```python
from build123d import *

# Parameters (mm, degrees)
BOSS_EXTRUDE1_DEPTH = 10
SKETCH2_R           = 2
CUT_EXTRUDE1_DEPTH  = 127.711975624
FILLET1_R           = 2
L_EK1_SCALE         = 2
L_EK2_SCALE         = 0.4


with BuildPart() as part:
    # Sketch1 → Boss-Extrude1 (new body)
    with BuildSketch(Plane(origin=(0, 0, 0), x_dir=(1, 0, 0), z_dir=(0, 1, 0))):
        with BuildLine():
            Line((5.38708673, 8.005739827), (-9.101800665, 4.12345415))
            Line((-9.101800665, 4.12345415), (7.721437267, -58.661724559))
            ThreePointArc((7.721437267, -58.661724559), (10.067992025, -70.873983123), (21.600150017, -75.52746682))
            Line((21.600150017, -75.52746682), (30.569895869, -119.624446982))
            Line((30.569895869, -119.624446982), (40.569895869, -119.624446982))
            Line((40.569895869, -119.624446982), (40.569895869, -39.624446982))
            Line((40.569895869, -39.624446982), (35.479571099, -42.800701652))
            Line((35.479571099, -42.800701652), (28.162650962, -57.029639761))
            Line((28.162650962, -57.029639761), (20.162650962, -55.994260173))
            Line((20.162650962, -55.994260173), (5.38708673, 8.005739827))
        make_face()
    extrude(amount=BOSS_EXTRUDE1_DEPTH)

    # Sketch2 → Cut-Extrude1 (cut, through all)
    with BuildSketch(Plane(origin=(0, 10, 0), x_dir=(1, 0, 0), z_dir=(0, 1, 0))):
        with Locations(Location((-4.202821179, 1.295027025, 0), (0, 0, 270))):
            Circle(SKETCH2_R)
    extrude(amount=-CUT_EXTRUDE1_DEPTH, mode=Mode.SUBTRACT)

    # Fillet1
    fillet1_edges = [part.edges().sort_by_distance(p)[0] for p in [
        (35.479571099, 5, 42.800701652),
        (40.569895869, 5, 39.624446982),
        (40.569895869, 5, 119.624446982),
        (30.569895869, 5, 119.624446982),
        (-9.101800665, 5, -4.12345415),
        (5.38708673, 5, -8.005739827),
    ]]
    fillet(fillet1_edges, radius=FILLET1_R)


with BuildPart() as part_1:
    # Ölçek1: scaled about (20.340725974, 5, 57.172914763)
    add(part.part.scale(L_EK1_SCALE).moved(Location((-20.340725974, -5, -57.172914763))))


with BuildPart() as part_2:
    # Ölçek2: scaled about (20.340725974, 5, 57.172914763)
    add(part_1.part.scale(L_EK2_SCALE).moved(Location((12.204435584, 3, 34.303748858))))


solid = part_2.part
```
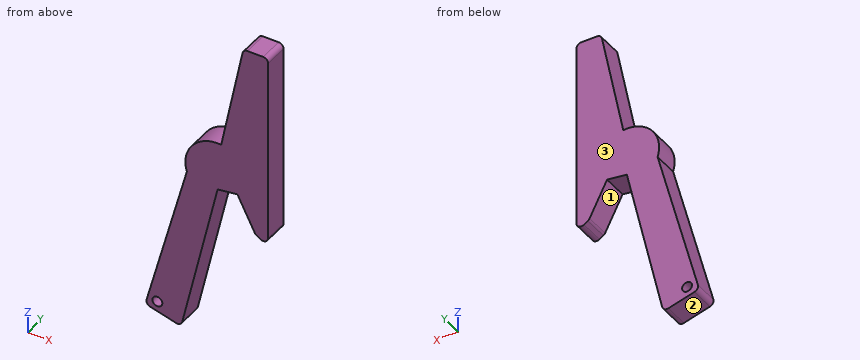
Here's how the part is built. I have some questions about the finished solid (model axes, mm). Face numbers are marked on the shaded views. Give positions to 0.01 mm unless a question says otherwise; leave off trailing zeros. Order: outer loops, then holes, each group sorted by start corner. A loop starts at its lowest first (then second) coordinate and runs counter-clockwise, first axis right, second up. Notation, with made-up numbers: M 54,26 L 78,26 A25 ccw 78,44 Z; hole C 22,-37.75 d6. An arc over 180 degrees is marked long. Use a Markdown table: item, result. Add a question column.
1. If we mould it in two halves opening along X, with no side actions, what happens to the marked faces 1, 2 and 3? For each: +X half, -X half, draft (parallel to the pull), parting line (faces both ways), or undercut.
2. For pin 1 Ø4 at (y, z) = (4.5, 16) entering from -X; pin 2 Ø4 at (y, z) = (4.5, 62.5) entering from -X; pin 3 Ø4 at (x, y) = (30, 8) entering from -Z, each with a flat end and sliding along its axis, tell me the tip position at first contact or that it passes through.
3. Suppose I cut it at A-A (y = 6.5). List the corners of the cut face in (x, z) for me, and give its area (3 significant figures).
4. Suppose I cut it at B-B (z = 48.5). List the corners of the cut face in (x, y) for me, and give its area (3 significant figures).
5. Suppose I cut it at C-C (x = 31). List the corners of the cut face in (y, z) for me, and give its area (3 significant figures).
6. Suppose I cut it at D-D (z = 22). List the corners of the cut face in (x, y) for me, and give its area (3 significant figures).
7. I need wall thicknesses on probe 1 along X at (y, z) = (6.25, 62); probe 2 along X at (y, z) = (7.5, 14); probe 3 along Z at (x, y) = (30, 6). Which ranges of each line are inside material? Lowest first, please. Write a range as from..to.
Results list:
| question | item | result |
|---|---|---|
| 1 | face 1 | undercut |
| 1 | face 2 | -X half |
| 1 | face 3 | draft |
| 2 | pin 1 | stops at x = -1.64 |
| 2 | pin 2 | stops at x = 9.75 |
| 2 | pin 3 | stops at z = 46.55 |
| 3 | outline | M -2.8,9.68 A1.6 ccw -1.67,7.72 L 6.78,5.46 A1.6 ccw 8.75,6.64 L 20.2,56.23 L 26.6,57.06 L 32.25,46.07 A1.6 ccw 32.83,45.44 L 34.08,44.66 A1.6 ccw 36.52,46.02 L 36.52,105.53 A1.6 ccw 34.92,107.13 L 29.83,107.13 A1.6 ccw 28.26,105.85 L 21.35,71.86 A10.4 ccw 10.25,58.36 Z; hole C 0.71,10.4 d3.2 |
| 3 | area | 1,430 mm² |
| 4 | outline | M 7.6,1 L 18.41,1 L 18.41,9 L 7.6,9 Z; M 31,1 L 36.52,1 L 36.52,9 L 31,9 Z |
| 4 | area | 131 mm² |
| 5 | outline | M 1,48.5 L 9,48.5 L 9,107.13 L 1,107.13 Z |
| 5 | area | 469 mm² |
| 6 | outline | M 0.5,1 L 12.3,1 L 12.3,9 L 0.5,9 Z |
| 6 | area | 94.4 mm² |
| 7 | probe 1 | x = 9.76..36.52 |
| 7 | probe 2 | x = -1.64..10.45 |
| 7 | probe 3 | z = 50.44..107.13 |
